The listing builds one solid part. Answer for the finished solid, in the listing's coordinates (mm). Face numbers are marked on the shaded views. A direction names the side the tool comes from. Round coordinates to 2 decimals unless told otherwise and drop trailing zeros. Loops run counter-clockwise (first coordinate to the right, second up) from the corner with the lowest first, then second, coordinate; pieces in that order, holes last. Notation, with made-up numbers: (27, 86) -> (68, 86) arc R27 cw to (68, 125) -> close; hole circle Ø3 at (69.5, 34). An arc over 180 degrees is marked (long way). One line per question, with ' | ' between items.
Autodesk Inventor part; units mm, degrees
ref_plane "Work Plane1" through (-14, 0, 0) normal (1, 0, 0) x (0, 0, -1)
ref_plane "YZ Plane" through (0, 0, 0) normal (1, 0, 0) x (0, 1, 0)
ref_plane "XZ Plane" through (0, 0, 0) normal (0, 1, 0) x (-1, 0, 0)
sketch "Sketch1" plane through (0, 0, 0) normal (0, 1, 0) x (-1, 0, 0)
  line L0 (0, 0) -> (28, 0)
  line L1 (28, 0) -> (28, -28)
  line L2 (28, -28) -> (0, -28)
  line L3 (0, -28) -> (0, 0)
  line L4 (24.125, -3.875) -> (3.875, -3.875)
  line L5 (3.875, -3.875) -> (3.875, -24.125)
  line L6 (3.875, -24.125) -> (24.125, -24.125)
  line L7 (24.125, -24.125) -> (24.125, -3.875)
  line L8 (24.125, -3.875) -> (3.875, -24.125) construction
  line L9 (3.875, -3.875) -> (24.125, -24.125) construction
  line L10 (0, 0) -> (28, -28) construction
  line L11 (28, 0) -> (0, -28) construction
  point P0 (14, -14)
  dimension "externo" = 28
  dimension "externo2" = 28
  dimension "interno" = 20.25
  dimension "interno2" = 20.25
extrude "principal" add sketch "Sketch1" along normal blind 80
sketch "Sketch2" plane through (-28, 80, -28) normal (-1, 0, 0) x (0, 0, 1)
  circle A0 centre (14, -8.7403) radius 1.75
  point P0 (28, -80)
  dimension "hueco_tornillo" = 3.5
extrude "hueco1" cut sketch "Sketch2" against normal blind 7.75
sketch "Sketch3" plane through (0, 80, 0) normal (1, 0, 0) x (0, 0, -1)
  circle A0 centre (14, -8.7403) radius 1.75
  circle A1 centre (14, -8.7403) radius 1.75
  point P0 (0, -80)
  dimension "hueco_tornillo_2" = 3.5
extrude "hueco2" cut sketch "Sketch3" against normal blind 7.75
fillet "hueco_Fillet" radius 0.5 2 edges at (-3.875, 71.2597, -12.25) (-24.125, 71.2597, -15.75)
sketch "Sketch4" plane through (0, 0, -28) normal (0, 0, -1) x (-1, 0, 0)
  line L0 (28, 0) -> (0, 0)
  line L1 (0, 0) -> (28, 0)
  line L2 (28, 0) -> (28, 5)
  line L3 (28, 5) -> (0, 5)
  line L4 (0, 5) -> (0, 0)
  line L5 (0, 5) -> (5, 5)
  line L6 (5, 5) -> (5, 10)
  line L7 (5, 10) -> (0, 10)
  line L8 (0, 10) -> (0, 5)
  line L9 (28, 5) -> (23, 5)
  line L10 (23, 5) -> (23, 10)
  line L11 (23, 10) -> (28, 10)
  line L12 (28, 10) -> (28, 5)
  point P0 (23, 5)
  point P1 (5, 5)
  dimension "lateral_ancho" = 28
  dimension "lateral_espesor" = 5
  dimension "lateral_refuerzo_1_ancho" = 5
  dimension "lateral_refuerzo_1_alto" = 5
  dimension "lateral_refuerzo_2_ancho" = 5
  dimension "lateral_refuerzo_2_alto" = 5
extrude "lateral" add sketch "Sketch4" along normal blind 70
sketch "Sketch5" plane through (0, 0, 0) normal (1, 0, 0) x (0, 0, -1)
  line L0 (0, 80) -> (28, 80)
  line L1 (28, 10) -> (28, 80)
  line L2 (28, 80) -> (28, 10)
  line L3 (28, 10) -> (83, 10)
  line L4 (83, 10) -> (28, 80)
  point P0 (0, 0)
  dimension "refuerzo" = 55
extrude "escuadra" add sketch "Sketch5" against normal blind 5
ref_plane "Work Plane1" through (-14, 0, 0) normal (1, 0, 0) x (0, 0, -1)
mirror "escuadra_Mirror" about plane through (-14, 0, 0) normal (1, 0, 0) of "escuadra"
sketch "Sketch6" plane through (-23, 5, -28) normal (0, 1, 0) x (1, 0, 0)
  circle A0 centre (9, 60) radius 1.75
  line L0 (0, 70) -> (18, 70)
  point P0 (23, -28)
  dimension "hueco_tornillo_lateral" = 3.5
  dimension "hueco_lateral_sep" = 10
extrude "hueco_lateral" cut sketch "Sketch6" against normal blind 5
ref_plane "Work Plane2" through (-5, 5, -14) normal (0, 0, -1) x (-1, 0, 0)
mirror "lateral_mirror" about plane through (-5, 5, -14) normal (0, 0, -1) of "escuadra", "escuadra_Mirror", "lateral", "hueco_lateral"
fillet "entrada_Fillet" radius 1.5 4 edges at (-24.125, 80, -14) (-14, 80, -3.875) (-3.875, 80, -14) (-14, 80, -24.125)
equation "\"externo2\" = externo"
equation "\"interno2\" = interno"
equation "\"hueco_profundidad\" = externo - interno"
equation "\"hueco_tornillo_2\" = hueco_tornillo"
equation "\"hueco_profundidad_2\" = hueco_profundidad"
equation "\"lateral_ancho\" = externo"
equation "\"lateral_refuerzo_1_ancho\" = lateral_espesor"
equation "\"lateral_refuerzo_1_alto\" = lateral_espesor"
equation "\"lateral_refuerzo_2_ancho\" = lateral_espesor"
equation "\"lateral_refuerzo_2_alto\" = lateral_espesor"
equation "\"d23\" = lateral_espesor"
equation "\"hueco_tornillo_lateral\" = hueco_tornillo"
equation "\"d27\" = lateral_espesor"
properties part number "SoportePrincipal"
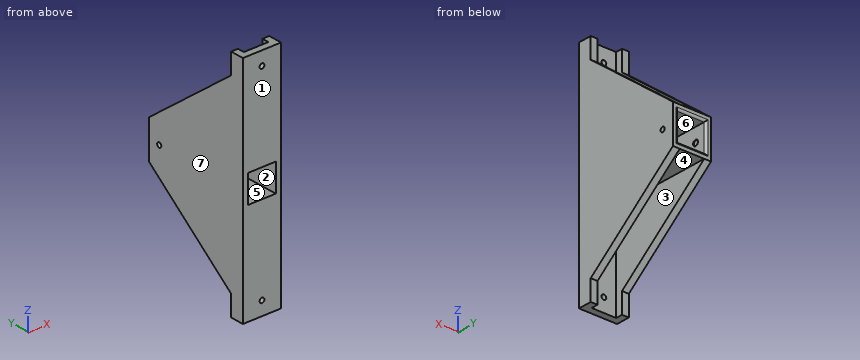
Q1. Given pin 1 Ø3 at (x, z) = (-24, -56.5) entering from +Y; pin 2 Ø3 at (x, y) = (-18, 64) entering from -Z; pin 3 Ø1.5 at (x, y) = (-24, 20) entering from -Z, each flat-ended and moving along its own axis, determine where each tip first touches the part or whether it passes through.
Numbers:
pin 1: y = 45.64 | pin 2: z = -28 | pin 3: z = -75.73
Q2. A cutting plane is placed at A-A on x = -14. Give the vertices of the cut face in (y, z) (3 decimals), plus the area to 3 significant figures.
Numbers:
outline: (0, -98) -> (5, -98) -> (5, -89.75) -> (0, -89.75) -> close; (0, -86.25) -> (5, -86.25) -> (5, -28) -> (80, -28) -> (80, -25.625) arc R1.5 ccw to (78.5, -24.125) -> (0, -24.125) -> close; (0, -3.875) -> (78.5, -3.875) arc R1.5 ccw to (80, -2.375) -> (80, 0) -> (5, 0) -> (5, 58.25) -> (0, 58.25) -> close; (0, 61.75) -> (5, 61.75) -> (5, 70) -> (0, 70) -> close | area: 1,280 mm^2
Q3. For the marked faces 1, 2 and 3, determine the directions among +Z, -Z, +X, -X, +Y, -Y from which every point of the face is accessible in a straight line to the end or side of a thin tool.
Numbers:
face 1: +Z, -Z, +X, -X, -Y | face 2: +Y, -Y | face 3: -Z, +Y
Q4. A cutting plane is placed at D-D on y = 7.5. Give the vertices of the cut face in (x, z) (3 decimals), plus the area to 3 significant figures.
Numbers:
outline: (-28, -98) -> (-23, -98) -> (-23, -28) -> (-5, -28) -> (-5, -98) -> (0, -98) -> (0, 70) -> (-5, 70) -> (-5, 0) -> (-23, 0) -> (-23, 70) -> (-28, 70) -> close; hole (-24.125, -24.125) -> (-3.875, -24.125) -> (-3.875, -3.875) -> (-24.125, -3.875) -> close | area: 1,770 mm^2
Q5. For a pull along Z with two mould halves and no side action, classify the marked faces 4, 5, 6 and 7 as pulls with the +Z half, pulls with the -Z half, needs draft (parallel to the pull), parting line crosses it, or undercut.
Numbers:
face 4: pulls with the -Z half | face 5: undercut | face 6: undercut | face 7: needs draft
Q6. Find the intervals of material crossed by line 1 (Z direction, x = -14, y = 3.25) (3 decimals); line 2 (Z direction, x = -8.5, y = 16) (3 decimals); line 3 (X direction, y = 2.9, z = -88), in increasing order. Write a range as from..to.
Numbers:
line 1: -98..-89.75, -86.25..-24.125, -3.875..58.25, 61.75..70 | line 2: -28..-24.125, -3.875..0 | line 3: -28..-15.75, -12.25..0
Q7. A cutting plane is placed at B-B on z = 60. Give the vertices of the cut face in (x, y), plus the area to 4 significant figures.
Numbers:
outline: (-28, 0) -> (-15.75, 0) -> (-15.75, 5) -> (-23, 5) -> (-23, 10) -> (-28, 10) -> close; (-12.25, 0) -> (0, 0) -> (0, 10) -> (-5, 10) -> (-5, 5) -> (-12.25, 5) -> close | area: 172.5 mm^2
Q8. A cutting plane is placed at C-C on z = -14. Give the vertices of the cut face in (x, y) (3 decimals), plus the area to 3 significant figures.
Numbers:
outline: (-28, 0) -> (-24.125, 0) -> (-24.125, 69.01) arc R0.5 ccw to (-24.625, 69.51) -> (-28, 69.51) -> close; (-28, 73.01) -> (-24.625, 73.01) arc R0.5 ccw to (-24.125, 73.51) -> (-24.125, 78.5) arc R1.5 ccw to (-25.625, 80) -> (-28, 80) -> close; (-3.875, 0) -> (0, 0) -> (0, 69.51) -> (-3.375, 69.51) arc R0.5 ccw to (-3.875, 69.01) -> close; (-3.875, 73.51) arc R0.5 ccw to (-3.375, 73.01) -> (0, 73.01) -> (0, 80) -> (-2.375, 80) arc R1.5 ccw to (-3.875, 78.5) -> close | area: 592 mm^2
